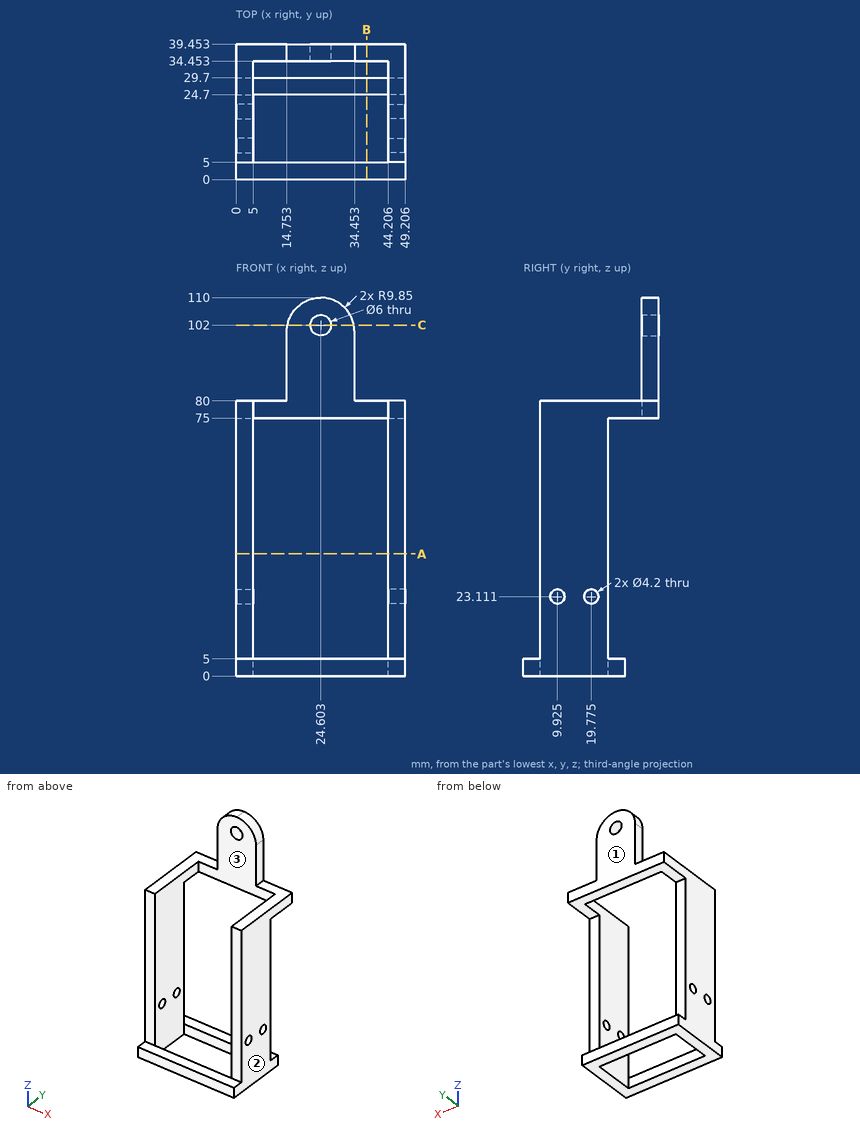
Source: three-view drawing plus pictorial views. Frame: mm from the lowest corner of the part. Coordinates: 2 decimals unless noted, no trailing zeros. Write each loop counter-clockwise with the first axis right and the second up, starting at its lowest first coordinate (ties: lowest second). Pieces come first, ordered by that corner, then holes. Notation, with made-up numbers: (47, 21.5) -> (75, 21.5) arc R23 cw to (75, 50.5) -> close; hole circle Ø6 at (17, 68). An arc over 180 degrees is marked (long way). Write each question's results on one line, items separated by ' | '.
Item 1: Section query A-A on z = 35.5. Return loops of the section in (x, y) (1 decimal).
Conclusion:
outline: (0, 5) -> (5, 5) -> (5, 24.7) -> (0, 24.7) -> close; (44.2, 5) -> (49.2, 5) -> (49.2, 24.7) -> (44.2, 24.7) -> close
Item 2: Section query C-C on z = 102. Return loops of the section in (x, y).
Conclusion:
outline: (14.93, 34.45) -> (21.6, 34.45) -> (21.6, 39.45) -> (14.93, 39.45) -> close; (27.6, 34.45) -> (34.28, 34.45) -> (34.28, 39.45) -> (27.6, 39.45) -> close
Item 3: Section query B-B on x = 38. Return loops of the section in (y, z).
Conclusion:
outline: (0, 0) -> (5, 0) -> (5, 5) -> (0, 5) -> close; (24.7, 0) -> (29.7, 0) -> (29.7, 5) -> (24.7, 5) -> close; (34.45, 75) -> (39.45, 75) -> (39.45, 80) -> (34.45, 80) -> close
Item 4: Mould query, pull axis X, two halves, no side actions, for the marked faces 1, 2 and 3. Classes: +X half, -X half, draft (parallel to the pull), parting line (faces both ways), or undercut.
Conclusion:
face 1: draft | face 2: +X half | face 3: undercut
Item 5: Pin query (flat end, axial travel): pin 1 Ø5.5 at (x, y) = (23.5, 28.5) entering from +Z; pin 2 Ø5.5 at (x, z) = (28.5, 2.5) entering from +Y; pin 3 Ø12 at (y, z) = (32.5, 90) entering from +X. Return the tip coordinate at first contact, or that it passes through.
Conclusion:
pin 1: stops at z = 5 | pin 2: stops at y = 29.7 | pin 3: stops at x = 34.45
Item 6: Material intervals for probe 1 along X at (y, z) = (17, 53.5) (1 decimal); probe 2 along Z at (x, y) = (45, 33); probe 3 along X at (y, z) = (36, 102), sorted ascending.
Conclusion:
probe 1: x = 0 to 5, 44.2 to 49.2 | probe 2: z = 75 to 80 | probe 3: x = 14.93 to 21.6, 27.6 to 34.28
